Verification items for the finished model (mm, model axes). Face numbers are marked on the shaded views. Give positions to 0.01 mm unless a question says otherwise; leave off trailing zeros. Order: outer loops, then holes, each group sorted by start corner. A loop starts at its lowest first (then second) coordinate and runs counter-clockwise, first axis right, second up. Notation, with made-up numbers: (32, 20.5) - (55, 20.5) arc R18 ccw to (55, 55.5) - close; hole circle Ø2 at (86, 18.5). An arc over 180 degrees is marked (long way). Answer as a JSON object with one key per item and string values. Group by question number.
(1) Section check A-A (x = 20). Count the separate pieces of the cut face and the enclosed holes in it, then the cut area to 3 significant figures.
(2) Section check B-B (y = 25). Record the boundary of the cut face in (x, z), then the cut area to 3 significant figures.
(3) Depth check by flat-ended pin: pin 1 Ø2 at (x, y) = (-2, 34) entering from +Z; pin 2 Ø0.9 at (x, z) = (11, 1) entering from -Y; pin 3 Ø3.5 at (x, y) = (-0.57, 27.49) entering from +Z. Enter the tip coordinate at first touch or a pass-through.
(4) Thickness scan on line 1 (X direction, y = 10, z = 2.45); line 2 (Z direction, x = -12, y = 34); line 3 (Y direction, x = -6, z = 2.1). Record the ranges inside material, lowest first.
(5) Mould release check, pull along X, two halves, no side actions. Record for the marked faces 1 and 2: +X half, -X half, draft (parallel to the pull), parting line (faces both ways), or undercut.
```python
from build123d import *

# Parameters (mm, degrees)
BOSS_EXTRU_1_DEPTH      = 3
ESQUISSE2_R             = 1.5
ENL_V_MAT_EXTRU_1_DEPTH = 48.507894081
ESQUISSE4_W             = 30
ESQUISSE4_H             = 24.796786232
ENL_V_MAT_EXTRU_3_DEPTH = 1.5
CONG_2_R                = 1


with BuildPart() as part:
    # Esquisse1 → Boss.-Extru.1 (new body)
    with BuildSketch(Plane.XY):
        with BuildLine():
            Line((-18, 2), (0, 2))
            Line((0, 2), (0, 0))
            Line((0, 0), (0, -3.563243554))
            ThreePointArc((0, -3.563243554), (5.005734949, -3.059001354), (9, 0))
            Line((9, 0), (6, 0))
            Line((6, 0), (6, 2))
            Line((6, 2), (22, 2))
            Line((22, 2), (22, 42))
            Line((22, 42), (-18, 42))
            Line((-18, 42), (-18, 2))
        make_face()
    extrude(amount=BOSS_EXTRU_1_DEPTH)

    # Esquisse2 → Enlèv. mat.-Extru.1 (cut, through all)
    with BuildSketch(Plane.XY.offset(3)):
        with Locations((-16, 37.48988726)):
            Circle(ESQUISSE2_R)
        with Locations((-10.857142857, 37.48988726)):
            Circle(ESQUISSE2_R)
        with Locations((-5.714285714, 37.48988726)):
            Circle(ESQUISSE2_R)
        with Locations((-0.571428571, 37.48988726)):
            Circle(ESQUISSE2_R)
        with Locations((4.571428571, 37.48988726)):
            Circle(ESQUISSE2_R)
        with Locations((9.714285714, 37.48988726)):
            Circle(ESQUISSE2_R)
        with Locations((14.857142857, 37.48988726)):
            Circle(ESQUISSE2_R)
        with Locations((20, 37.48988726)):
            Circle(ESQUISSE2_R)
        with Locations((-10.857142857, 32.48988726)):
            Circle(ESQUISSE2_R)
        with Locations((-5.714285714, 32.48988726)):
            Circle(ESQUISSE2_R)
        with Locations((-0.571428571, 32.48988726)):
            Circle(ESQUISSE2_R)
        with Locations((4.571428571, 32.48988726)):
            Circle(ESQUISSE2_R)
        with Locations((9.714285714, 32.48988726)):
            Circle(ESQUISSE2_R)
        with Locations((14.857142857, 32.48988726)):
            Circle(ESQUISSE2_R)
        with Locations((-10.857142857, 27.48988726)):
            Circle(ESQUISSE2_R)
        with Locations((-5.714285714, 27.48988726)):
            Circle(ESQUISSE2_R)
        with Locations((-0.571428571, 27.48988726)):
            Circle(ESQUISSE2_R)
        with Locations((4.571428571, 27.48988726)):
            Circle(ESQUISSE2_R)
        with Locations((9.714285714, 27.48988726)):
            Circle(ESQUISSE2_R)
        with Locations((14.857142857, 27.48988726)):
            Circle(ESQUISSE2_R)
        with Locations((-10.857142857, 22.48988726)):
            Circle(ESQUISSE2_R)
        with Locations((-5.714285714, 22.48988726)):
            Circle(ESQUISSE2_R)
        with Locations((-0.571428571, 22.48988726)):
            Circle(ESQUISSE2_R)
        with Locations((4.571428571, 22.48988726)):
            Circle(ESQUISSE2_R)
        with Locations((9.714285714, 22.48988726)):
            Circle(ESQUISSE2_R)
        with Locations((14.857142857, 22.48988726)):
            Circle(ESQUISSE2_R)
        with Locations((-10.857142857, 17.48988726)):
            Circle(ESQUISSE2_R)
        with Locations((-5.714285714, 17.48988726)):
            Circle(ESQUISSE2_R)
        with Locations((-0.571428571, 17.48988726)):
            Circle(ESQUISSE2_R)
        with Locations((4.571428571, 17.48988726)):
            Circle(ESQUISSE2_R)
        with Locations((9.714285714, 17.48988726)):
            Circle(ESQUISSE2_R)
        with Locations((14.857142857, 17.48988726)):
            Circle(ESQUISSE2_R)
        with Locations((-10.857142857, 12.48988726)):
            Circle(ESQUISSE2_R)
        with Locations((-5.714285714, 12.48988726)):
            Circle(ESQUISSE2_R)
        with Locations((-0.571428571, 12.48988726)):
            Circle(ESQUISSE2_R)
        with Locations((4.571428571, 12.48988726)):
            Circle(ESQUISSE2_R)
        with Locations((9.714285714, 12.48988726)):
            Circle(ESQUISSE2_R)
        with Locations((14.857142857, 12.48988726)):
            Circle(ESQUISSE2_R)
        with Locations((-10.857142857, 7.48988726)):
            Circle(ESQUISSE2_R)
        with Locations((-5.714285714, 7.48988726)):
            Circle(ESQUISSE2_R)
        with Locations((-0.571428571, 7.48988726)):
            Circle(ESQUISSE2_R)
        with Locations((4.571428571, 7.48988726)):
            Circle(ESQUISSE2_R)
        with Locations((9.714285714, 7.48988726)):
            Circle(ESQUISSE2_R)
        with Locations((14.857142857, 7.48988726)):
            Circle(ESQUISSE2_R)
        with Locations((-16, 32.48988726)):
            Circle(ESQUISSE2_R)
        with Locations((-16, 27.48988726)):
            Circle(ESQUISSE2_R)
        with Locations((-16, 22.48988726)):
            Circle(ESQUISSE2_R)
        with Locations((-16, 17.48988726)):
            Circle(ESQUISSE2_R)
        with Locations((-16, 12.48988726)):
            Circle(ESQUISSE2_R)
        with Locations((-16, 7.48988726)):
            Circle(ESQUISSE2_R)
        with Locations((20, 32.48988726)):
            Circle(ESQUISSE2_R)
        with Locations((20, 27.48988726)):
            Circle(ESQUISSE2_R)
        with Locations((20, 22.48988726)):
            Circle(ESQUISSE2_R)
        with Locations((20, 17.48988726)):
            Circle(ESQUISSE2_R)
        with Locations((20, 12.48988726)):
            Circle(ESQUISSE2_R)
        with Locations((20, 7.48988726)):
            Circle(ESQUISSE2_R)
    extrude(amount=-ENL_V_MAT_EXTRU_1_DEPTH, mode=Mode.SUBTRACT)

    # Esquisse4 → Enlèv. mat.-Extru.3 (cut)
    with BuildSketch(Plane.XY.offset(3)):
        with Locations((2, 22)):
            Rectangle(ESQUISSE4_W, ESQUISSE4_H)
    extrude(amount=-ENL_V_MAT_EXTRU_3_DEPTH, mode=Mode.SUBTRACT)

    # Congé2
    cong_2_edges = [part.edges().sort_by_distance(p)[0] for p in [
        (0, -3.563243554, 1.5),
    ]]
    fillet(cong_2_edges, radius=CONG_2_R)


solid = part.part
```
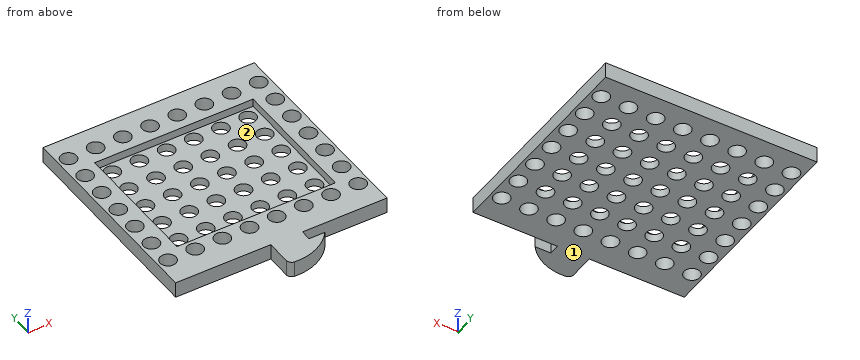
Solutions:
{
 "1": {"separate pieces": "8", "enclosed holes": "0", "area": "57.0 mm2"},
 "2": {"outline": "(-18, 0) - (22, 0) - (22, 3) - (17, 3) - (17, 1.5) - (-13, 1.5) - (-13, 3) - (-18, 3) - close", "area": "75.0 mm2"},
 "3": {"pin 1": "stops at z = 3", "pin 2": "stops at y = 2", "pin 3": "stops at z = 1.5"},
 "4": {"line 1": "x = -18 to -13, 17 to 22", "line 2": "z = 0 to 1.5", "line 3": "y = 2 to 6.02, 8.96 to 9.6, 34.4 to 36.02, 38.96 to 42"},
 "5": {"face 1": "draft", "face 2": "undercut"}
}
